CAD build for the part. Positions are in the model's coordinates, mm. Round coordinates to 2 decimals unless told otherwise and drop trailing zeros. Loops run counter-clockwise (first coordinate to the right, second up) from the corner with the lowest first, then second, coordinate; pieces in that order, holes last.
Autodesk Inventor part; units mm, degrees
ref_plane "YZ Plane" through (0, 0, 0) normal (1, 0, 0) x (0, 1, 0)
ref_plane "XZ Plane" through (0, 0, 0) normal (0, 1, 0) x (-1, 0, 0)
ref_plane "XY Plane" through (0, 0, 0) normal (0, 0, 1) x (1, 0, 0)
sketch "Sketch1" plane through (0, 0, 0) normal (0, 1, 0) x (-1, 0, 0)
  line L0 (0, 0) -> (19.05, 0)
  line L1 (19.05, 0) -> (19.05, 19.05)
  line L2 (19.05, 19.05) -> (0, 19.05)
  line L3 (0, 19.05) -> (0, 0)
  line L4 (1.778, 17.272) -> (17.272, 17.272)
  line L5 (17.272, 17.272) -> (17.272, 1.778)
  line L6 (17.272, 1.778) -> (1.778, 1.778)
  line L7 (1.778, 1.778) -> (1.778, 17.272)
  dimension "MastWidth" = 19.05
  dimension "d1" = 19.05
  dimension "d2" = 1.778
  dimension "d3" = 1.778
  dimension "d4" = 1.778
  dimension "d5" = 1.778
extrude "Extrusion1" add sketch "Sketch1" along normal blind 1524
sketch "Sketch2" plane through (0, 0, 0) normal (0, -1, 0) x (1, 0, 0)
  line L0 (-17.272, 1.778) -> (-17.272, 17.272)
  line L1 (-17.272, 17.272) -> (-1.778, 17.272)
  line L2 (-1.778, 17.272) -> (-1.778, 1.778)
  line L3 (-1.778, 1.778) -> (-17.272, 1.778)
  line L4 (0, 0) -> (-19.05, 0)
  line L5 (0, 19.05) -> (0, 0)
  line L6 (-19.05, 19.05) -> (0, 19.05)
  line L7 (-19.05, 0) -> (-19.05, 19.05)
  line L8 (-19.05, 9.525) -> (0, 9.525)
  line L9 (-9.525, 19.05) -> (-9.525, 0)
sketch "Sketch3" plane through (-19.05, 0, 19.05) normal (0, 0, 1) x (1, 0, 0)
  line L0 (19.05, 1524) -> (0, 1524)
  line L1 (0, 0) -> (0, 1524)
  line L2 (0, 0) -> (19.05, 0)
  line L3 (19.05, 0) -> (19.05, 1524)
  line L4 (7.0234, 1484.4913) -> (20.0256, 1484.4913) construction
  line L5 (20.0256, 1484.4913) -> (20.0256, 1481.3149) construction
  line L6 (20.0256, 1481.3149) -> (7.0234, 1481.3149) construction
  line L7 (7.0234, 1481.3149) -> (7.0234, 1484.4913) construction
sketch "Sketch4" plane through (-19.05, 0, 19.05) normal (0, 0, 1) x (1, 0, 0)
  circle A0 centre (9.525, 88.7067) radius 6.35
  dimension "d8" = 12.7
extrude "Extrusion2" cut sketch "Sketch4" against normal blind 6.35
equation "\"d1\" = MastWidth"
equation "\"d3\" = d2"
equation "\"d4\" = d2"
equation "\"d5\" = d2"
properties part number "Robot-Mast" material "Aluminum-6061"
Item 1: Cut at C-C, the plane x = -12.5. Give the cut face in (y, z).
Answers follow:
outline: (0, 0) - (1524, 0) - (1524, 1.78) - (0, 1.78) - close; (0, 17.27) - (83.1, 17.27) - (83.1, 19.05) - (0, 19.05) - close; (94.32, 17.27) - (1524, 17.27) - (1524, 19.05) - (94.32, 19.05) - close
Item 2: Probe line 1 (Z direction, x = -9.75, y = 1443); line 2 (X direction, y = 254, z = 16.25); line 3 (Y direction, x = -6, z = 18.25). List the from-to ranges inside material, lowest first.
Answers follow:
line 1: z = 0 to 1.78, 17.27 to 19.05
line 2: x = -19.05 to -17.27, -1.78 to 0
line 3: y = 0 to 83.42, 93.99 to 1524
Item 3: Flat gauge pins, fed straight in: P1, Ø1, axis at y = 1137, z = 9, coming from the +X side; P2, Ø2, axis at x = -3.5, z = 3.5, coming from the -Y side. Where does each tip first touch, or does it go through?
Answers follow:
P1: stops at x = 0
P2: passes through
Item 4: Cut at B-B, the plane y = 1110. Give the cut face in (x, z).
Answers follow:
outline: (-19.05, 0) - (0, 0) - (0, 19.05) - (-19.05, 19.05) - close; hole (-17.27, 1.78) - (-1.78, 1.78) - (-1.78, 17.27) - (-17.27, 17.27) - close
Item 5: Cut at A-A, the plane z = 8.5. Give the cut face in (x, y).
Answers follow:
outline: (-19.05, 0) - (-17.27, 0) - (-17.27, 1524) - (-19.05, 1524) - close; (-1.78, 0) - (0, 0) - (0, 1524) - (-1.78, 1524) - close
